Model file for the job. Use its own axes, mm. A direction names the side the tool comes from. Round coordinates to 2 decimals unless told otherwise and drop trailing zeros. Loops run counter-clockwise (first coordinate to the right, second up) from the corner with the lowest first, then second, coordinate; pieces in that order, holes last.
from build123d import *

# Parameters (mm, degrees)
F0_R     = 40
F1_DEPTH = 120
F2_R     = 2.5
F3_DEPTH = 25
F4_DEPTH = 30


with BuildPart() as f1:
    # F0 (on Top) → F1 (new body)
    with BuildSketch(Plane.XY):
        Circle(F0_R)
    extrude(amount=F1_DEPTH)

    # F2 (on face) → F3 (join)
    with BuildSketch(Plane(origin=(0, 0, 0), x_dir=(1, 0, 0), z_dir=(0, 0, -1))):
        Circle(F2_R)
    extrude(amount=F3_DEPTH)

    # F2 (on face) → F4 (join)
    with BuildSketch(Plane(origin=(0, 0, 0), x_dir=(1, 0, 0), z_dir=(0, 0, -1))):
        Circle(F2_R)
    extrude(amount=F4_DEPTH)


solid = f1.part
Q1. Tool access for faces 1 (the face through (-1, 1, 120)), 2 (the face through (-0.54, 2.44, -14.79)): list every direction of +Z, -Z, +X, -X, +Y, -Y with a clear straight run to the whole face (end or side of a thin tool).
Q2. Slice it at A-A on y = 0. Give the cut face in (x, z).
Q3. Flat gauge pins, fed straight in: P1, Ø4, axis at y = 22.5, z = 38, coming from the -X side; P2, Ø8, axis at x = -21.5, z = 34, coming from the -Y side; P3, Ø3, axis at x = -22, z = 33, coming from the +Y side. Where does each tip first touch, or does it go through?
Q4. Slice it at C-C on z = 80. Give the cut face in (x, y), plus the area to 3 significant figures.
Q5. Probe line 1 (Z direction, x = 18, y = 26.5); line 2 (Y direction, x = -0.5, z = 101); line 3 (Y direction, x = 5, z = 20). List the from-to ranges inside material, lowest first.
Q6. Slice it at D-D on y = -32.5. Give the cut face in (x, z), plus the area to 3 significant figures.
Reply:
1. face 1: +Z, +X, -X, +Y, -Y
1. face 2: -Z
2. outline: (-40, 0) - (-2.5, 0) - (-2.5, -30) - (2.5, -30) - (2.5, 0) - (40, 0) - (40, 120) - (-40, 120) - close
3. P1: stops at x = -34.35
3. P2: stops at y = -35.97
3. P3: stops at y = 34.35
4. outline: circle Ø80 at (0, 0)
4. area: 5,030 mm2
5. line 1: z = 0 to 120
5. line 2: y = -40 to 40
5. line 3: y = -39.69 to 39.69
6. outline: (-23.32, 0) - (23.32, 0) - (23.32, 120) - (-23.32, 120) - close
6. area: 5,600 mm2
